from build123d import *

# Parameters (mm, degrees)
BOSS_EXTRUDE1_DEPTH = 46
SKETCH3_R           = 6.5
BOSS_EXTRUDE2_DEPTH = 10
CUT_EXTRUDE7_DEPTH  = 6
CIRPATTERN1_COUNT   = 4
SKETCH12_R          = 6.5
CUT_EXTRUDE8_DEPTH  = 30
CUT_EXTRUDE9_DEPTH  = 10
SKETCH14_R          = 1.705
CUT_EXTRUDE10_DEPTH = 12.5


with BuildPart() as part:
    # Sketch1 → Boss-Extrude1 (new body)
    with BuildSketch(Plane.XY):
        with BuildLine():
            Line((-5.05, 9.05), (5.05, 9.05))
            ThreePointArc((5.05, 9.05), (7.878427125, 7.878427125), (9.05, 5.05))
            Line((9.05, 5.05), (9.05, -5.05))
            ThreePointArc((9.05, -5.05), (7.878427125, -7.878427125), (5.05, -9.05))
            Line((5.05, -9.05), (-5.05, -9.05))
            ThreePointArc((-5.05, -9.05), (-7.878427125, -7.878427125), (-9.05, -5.05))
            Line((-9.05, -5.05), (-9.05, 5.05))
            ThreePointArc((-9.05, 5.05), (-7.878427125, 7.878427125), (-5.05, 9.05))
        make_face()
    extrude(amount=BOSS_EXTRUDE1_DEPTH)

    # Sketch3 → Boss-Extrude2 (add)
    with BuildSketch(Plane.XY.offset(46)):
        Polygon((-5, -7), (5, -7), (7, -5), (7, 5), (5, 7), (-5, 7), (-7, 5), (-7, -5), align=None)
        Circle(SKETCH3_R, mode=Mode.SUBTRACT)
    extrude(amount=BOSS_EXTRUDE2_DEPTH)

    # Sketch11 → Cut-Extrude7 (cut)
    with BuildSketch(Plane.XY.offset(56)):
        Polygon((0, 0), (7, 0.45), (7, -0.45), align=None)
    cut_extrude7 = extrude(amount=-CUT_EXTRUDE7_DEPTH, mode=Mode.SUBTRACT)

    # CirPattern1: Cut-Extrude7 ×4 about axis
    cirpattern1_axis = Axis((0, 0, 56), (0, 0, -1))
    for i in range(1, CIRPATTERN1_COUNT):
        add(cut_extrude7.rotate(cirpattern1_axis, i * 360 / CIRPATTERN1_COUNT), mode=Mode.SUBTRACT)

    # Sketch12 → Cut-Extrude8 (cut)
    with BuildSketch(Plane.XY.offset(46)):
        with Locations((0, 0.192488852)):
            Circle(SKETCH12_R)
    extrude(amount=-CUT_EXTRUDE8_DEPTH, mode=Mode.SUBTRACT)

    # Sketch13 → Cut-Extrude9 (cut)
    with BuildSketch(Plane.XY):
        with BuildLine():
            Line((-2.5, 0), (-2.5, 9.05))
            Line((-2.5, 9.05), (2.5, 9.05))
            Line((2.5, 9.05), (2.5, 0))
            ThreePointArc((2.5, 0), (0, -2.5), (-2.5, 0))
        make_face()
    extrude(amount=CUT_EXTRUDE9_DEPTH, mode=Mode.SUBTRACT)

    # Sketch14 → Cut-Extrude10 (cut, symmetric)
    with BuildSketch(Plane(origin=(0, 0, 0), x_dir=(0, 0, -1), z_dir=(1, 0, 0))):
        with Locations((-4.963568093, 5.105)):
            Circle(SKETCH14_R)
    extrude(amount=CUT_EXTRUDE10_DEPTH, both=True, mode=Mode.SUBTRACT)


solid = part.part
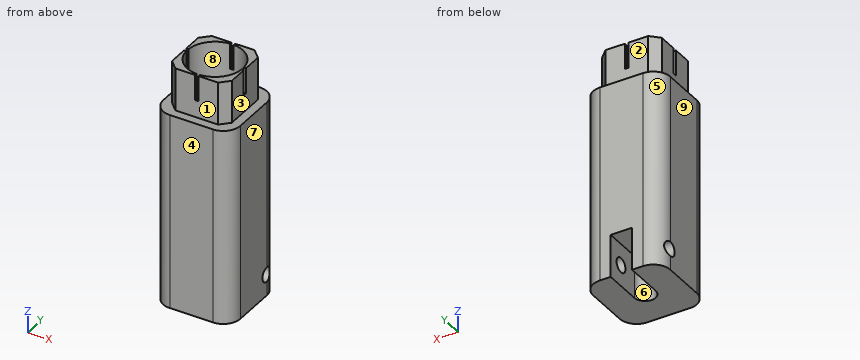
The model under review builds one solid part; all positions refer to its coordinate system, in mm. Face numbers are marked on the shaded views. A direction names the side the tool comes from. Coordinates: 2 decimals unless noted, no trailing zeros. Write each loop counter-clockwise with the first axis right and the second up, starting at its lowest first coordinate (ties: lowest second). Pieces come first, ordered by that corner, then holes. Notation, with made-up numbers: (-23.5, 36) -> (-3.5, 36) arc R31 ccw to (-3.5, 60) -> close; hole circle Ø6 at (-36, 38.5). An arc over 180 degrees is marked (long way). Answer in a Markdown table with one row per item.
1. For the marked faces 1, 2, 3, 4 and 5, list the 3-axis set-ups (+Z, -Z, +X, -X, +Y, -Y) from which the entire face can be reached by the end or side of a thin tool; tool diameter is ignored.
Answers below:
| item | result |
|---|---|
| face 1 | +Z, +X, -X, -Y |
| face 2 | +Z, +X, -X, +Y |
| face 3 | +Z, +X, +Y, -Y |
| face 4 | +Z, -Z, +X, -X, -Y |
| face 5 | +Z, -Z, -X, +Y |
2. Wall thickness on probe 1 along Y at (x, z) = (0, 49.5); probe 2 along Y at (x, z) = (0, 31); probe 3 along Z at (x, y) = (-3.25, 5.25): over which ranges is each line inside the solid? List them lowest first. Write a range as [from, to].
Answers below:
| item | result |
|---|---|
| probe 1 | y = [-7, -6.5], [6.5, 7] |
| probe 2 | y = [-9.05, -6.31], [6.69, 9.05] |
| probe 3 | z = [0, 3.26], [6.66, 16] |
3. We need section C-C, the plane y = 1.5. State the section outline as (x, z) points, and give its area (3 significant figures).
Answers below:
| item | result |
|---|---|
| outline | (-9.05, 0) -> (-2.5, 0) -> (-2.5, 10) -> (2.5, 10) -> (2.5, 0) -> (9.05, 0) -> (9.05, 46) -> (7, 46) -> (7, 56) -> (6.32, 56) -> (6.32, 46) -> (6.37, 46) -> (6.37, 16) -> (-6.37, 16) -> (-6.37, 46) -> (-6.32, 46) -> (-6.32, 56) -> (-7, 56) -> (-7, 46) -> (-9.05, 46) -> close |
| area | 414 mm^2 |
4. Draft analysis for pull direction X (two halves, no side actions). For the marked faces 6, 7, 8 and 9, state which applies: +X half, -X half, draft (parallel to the pull), parting line (faces both ways), or undercut.
Answers below:
| item | result |
|---|---|
| face 6 | undercut |
| face 7 | +X half |
| face 8 | undercut |
| face 9 | -X half |
5. Clearance check with flat-ended pins moving along their axes: pin 1 Ø1 at (x, y) = (-4, 3) entering from +Z; pin 2 Ø3 at (x, z) = (2, 51.5) entering from -Y; pin 3 Ø0.6 at (x, y) = (0, 6.5) entering from +Z. State where each tip first meets the part, or that it passes through.
Answers below:
| item | result |
|---|---|
| pin 1 | stops at z = 16 |
| pin 2 | stops at y = -7 |
| pin 3 | stops at z = 50 |
6. We need section A-A, the plane z = 52.5. State the section outline as (x, y) points, and give its area (3 significant figures).
Answers below:
| item | result |
|---|---|
| outline | (-7, -5) -> (-5, -7) -> (-0.45, -7) -> (-0.42, -6.49) arc R6.5 cw to (-6.49, -0.42) -> (-7, -0.45) -> close; (-7, 0.45) -> (-6.49, 0.42) arc R6.5 cw to (-0.42, 6.49) -> (-0.45, 7) -> (-5, 7) -> (-7, 5) -> close; (0.42, -6.49) -> (0.45, -7) -> (5, -7) -> (7, -5) -> (7, -0.45) -> (6.49, -0.42) arc R6.5 cw to start; (0.42, 6.49) arc R6.5 cw to (6.49, 0.42) -> (7, 0.45) -> (7, 5) -> (5, 7) -> (0.45, 7) -> close |
| area | 53.5 mm^2 |
7. We need section D-D, the plane z = 24. State the section outline as (x, y) points, and give its area (3 significant figures).
Answers below:
| item | result |
|---|---|
| outline | (-9.05, -5.05) arc R4 ccw to (-5.05, -9.05) -> (5.05, -9.05) arc R4 ccw to (9.05, -5.05) -> (9.05, 5.05) arc R4 ccw to (5.05, 9.05) -> (-5.05, 9.05) arc R4 ccw to (-9.05, 5.05) -> close; hole circle Ø13 at (0, 0.19) |
| area | 181 mm^2 |
8. We need section B-B, the plane z = 15.5. State the section outline as (x, y) points, and give its area (3 significant figures).
Answers below:
| item | result |
|---|---|
| outline | (-9.05, -5.05) arc R4 ccw to (-5.05, -9.05) -> (5.05, -9.05) arc R4 ccw to (9.05, -5.05) -> (9.05, 5.05) arc R4 ccw to (5.05, 9.05) -> (-5.05, 9.05) arc R4 ccw to (-9.05, 5.05) -> close |
| area | 314 mm^2 |
